Here's how the part is built. I have some questions about the finished solid (model axes, mm). Face numbers are marked on the shaded views. A direction names the side the tool comes from. Coordinates: 2 decimals unless noted, no trailing zeros. Write each loop counter-clockwise with the first axis right and the second up, starting at its lowest first coordinate (ties: lowest second). Pieces come first, ordered by that corner, then holes. Notation, with made-up numbers: M -23.5,81 L -6.5,81 A32 cw -6.5,110 Z; hole C 11.5,73 d11. An arc over 180 degrees is marked long. Use a Markdown table: item, result.
```python
from build123d import *

# Parameters (mm, degrees)
F0_W        = 14
F0_H        = 2
F1_DEPTH    = 15.5
F2_W        = 14
F2_H        = 3
F2_H_2      = 2
F3_DEPTH    = 4
F4_SIZE2    = 2
F4_SIZE     = 3
F5_T1_DEPTH = 24.5
F5_T3_DEPTH = 6
F7_DEPTH    = 15


# Not quite as in the source:
# - a fillet or chamfer that OpenCascade refuses, or shapes differently, is made with other operations: its cross-section is extruded or revolved along the edge and cut away or added


with BuildPart() as f1:
    # F0 (on Top) → F1 (new body)
    with BuildSketch(Plane.XY):
        Rectangle(F0_W, F0_H)
    extrude(amount=F1_DEPTH)

    # F2 (on face) → F3 (join)
    with BuildSketch(Plane.XY.offset(15.5)):
        with Locations((0, 2.5)):
            Rectangle(F2_W, F2_H)
        Rectangle(F2_W, F2_H_2)
    extrude(amount=F3_DEPTH)

    # F4
    f4_edges = [f1.edges().sort_by_distance(p)[0] for p in [
        (0, 4, 19.5),
    ]]
    f4_side = f1.faces().sort_by_distance((0, 4, 17.5))[0]
    chamfer(f4_edges, length=F4_SIZE, length2=F4_SIZE2, reference=f4_side)

    # F5: fillet of radius 1 on 4 edges, made by hand

    # F5_s2 → F5_t1 (cut)
    with BuildSketch(Plane.XY.offset(-2.5)):
        with BuildLine():
            add(Edge.make_bspline(
                [(-7, 0), (-7, -1), (-6, -1)],
                knots=[0, 0, 0, 1, 1, 1], degree=2, weights=[1, 1, 1]))
            Line((-6, -1), (-7, -1))
            Line((-7, -1), (-7, 0))
        make_face()
        with BuildLine():
            add(Edge.make_bspline(
                [(7, 0), (7, -1), (6, -1)],
                knots=[0, 0, 0, 1, 1, 1], degree=2, weights=[1, 1, 1]))
            Line((6, -1), (7, -1))
            Line((7, -1), (7, 0))
        make_face()
    extrude(amount=F5_T1_DEPTH, mode=Mode.SUBTRACT)

    # F5_s4 → F5_t3 (cut)
    with BuildSketch(Plane.XY.offset(13)):
        with BuildLine():
            add(Edge.make_bspline(
                [(-6, 4), (-7, 4), (-7, 3)],
                knots=[0, 0, 0, 1, 1, 1], degree=2, weights=[1, 1, 1]))
            Line((-7, 3), (-7, 4))
            Line((-7, 4), (-6, 4))
        make_face()
        with BuildLine():
            add(Edge.make_bspline(
                [(6, 4), (7, 4), (7, 3)],
                knots=[0, 0, 0, 1, 1, 1], degree=2, weights=[1, 1, 1]))
            Line((7, 3), (7, 4))
            Line((7, 4), (6, 4))
        make_face()
    extrude(amount=F5_T3_DEPTH, mode=Mode.SUBTRACT)

    # F6 (on face) → F7 (join)
    with BuildSketch(Plane(origin=(0, 0, 0), x_dir=(1, 0, 0), z_dir=(0, 0, -1))):
        with BuildLine():
            Line((-1, 1), (1, 1))
            ThreePointArc((1, 1), (0, 2), (-1, 1))
        make_face()
        with BuildLine():
            Line((5, 1), (3, 1))
            ThreePointArc((3, 1), (4, 0), (5, 1))
        make_face()
        with BuildLine():
            ThreePointArc((5, 1), (4, 2), (3, 1))
            Line((3, 1), (5, 1))
        make_face()
        with BuildLine():
            Line((-5, 1), (-3, 1))
            ThreePointArc((-3, 1), (-4, 2), (-5, 1))
        make_face()
    extrude(amount=-F7_DEPTH)


solid = f1.part
```
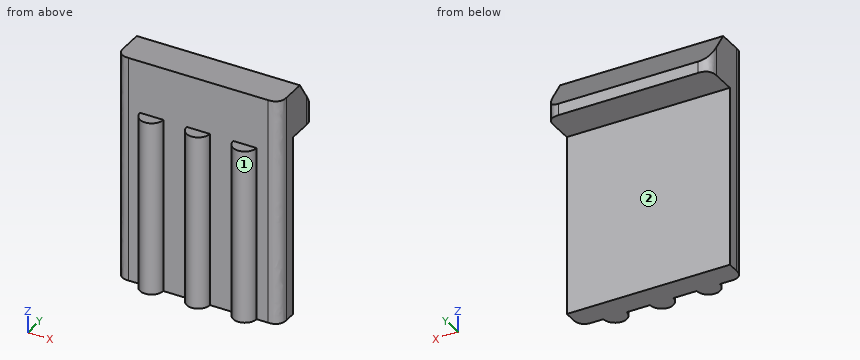
1. Suppose I cut it at B-B on x = 0. Write out the boundary of the cut face in (y, z).
Answers follow:
| item | result |
|---|---|
| outline | M -2,0 L 1,0 L 1,15.5 L 4,15.5 L 4,16.5 L 2,19.5 L -1,19.5 L -1,15 L -2,15 Z |
2. Suppose I cut it at A-A on x = 1.5. Write out the boundary of the cut face in (y, z), and give its area (3 significant figures).
Answers follow:
| item | result |
|---|---|
| outline | M -1,0 L 1,0 L 1,15.5 L 4,15.5 L 4,16.5 L 2,19.5 L -1,19.5 Z |
| area | 48.0 mm2 |
3. Suppose I cut it at C-C on y = 2.75. Write out the boundary of the cut face in (x, z) (3 decimals), and give its area (4 significant figures).
Answers follow:
| item | result |
|---|---|
| outline | M -7,15.5 L 7,15.5 L 7,18.375 L -7,18.375 Z |
| area | 40.25 mm2 |
4. Will these pins go through, and if not, where does the flat tip stop? pin 1 Ø1 at (x, y) = (-1.5, 3.5) entering from -Z; pin 2 Ø1.5 at (x, y) = (-5.5, 3.5) entering from +Z (3 decimals); pin 3 Ø0.5 at (x, y) = (-3.5, -1.5) entering from +Z.
Answers follow:
| item | result |
|---|---|
| pin 1 | stops at z = 15.5 |
| pin 2 | stops at z = 18.375 |
| pin 3 | stops at z = 15 |
5. I need wall thicknesses on probe 1 along X at (y, z) = (-1.25, 3.5); probe 2 along Y at (x, z) = (2.5, 4.5); probe 3 along Z at (x, y) = (-0.5, 1.5). Which ranges of each line are inside material? Lowest first, please.
Answers follow:
| item | result |
|---|---|
| probe 1 | x = -4.97 to -3.03, -0.97 to 0.97, 3.03 to 4.97 |
| probe 2 | y = -1 to 1 |
| probe 3 | z = 15.5 to 19.5 |
6. Which directions (+Z, -Z, +X, -X, +Y, -Y) give clear straight access to the entire face, cutting with the end or side of a thin tool? Please do the marked faces 1 and 2.
Answers follow:
| item | result |
|---|---|
| face 1 | +Z, -Z, -Y |
| face 2 | -Z, +X, -X, +Y |
